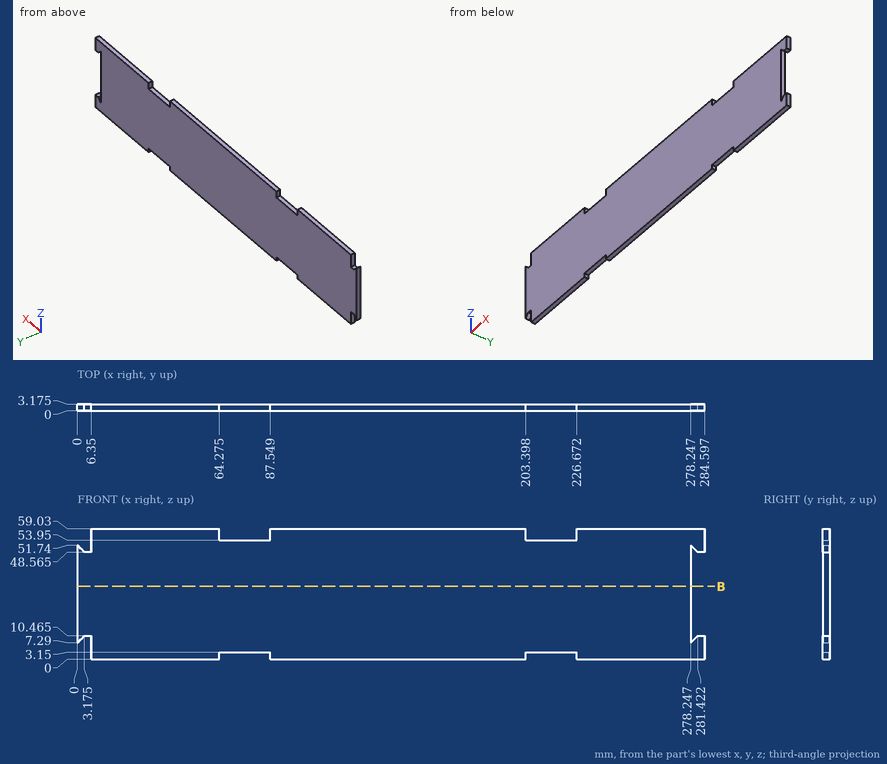
Could you check a few things on this drawing? It's one solid part, dimensions in mm from its lowest x, y, z. Coordinates: 2 decimals unless noted, no trailing zeros. Loops run counter-clockwise (first coordinate to the right, second up) from the corner with the lowest first, then second, coordinate; pieces in that order, holes last. Notation, with made-up numbers: (-14.5, 67) - (10.5, 67) arc R14 cw to (10.5, 79) - close; hole circle Ø11 at (40, 33.5). An arc over 180 degrees is marked (long way). Answer as a JSON object with one key per item and string values. Group by question number.
Item 1: For pin 1 (1 mm diameter, centred on x = 5.5, y = 1, fed in from +Z) (1 decimal); pin 2 (1 mm diameter, centred on y = 1, z = 55, fed in from -X); pin 3 (1.6 mm diameter, centred on x = 5, y = 2, fed in from -Z) (1 decimal), each with a flat end and sliding along its axis, tell me the tip position at first contact or that it passes through.
Item 2: If I drill on L1, parallel to X at y = 2.5, z = 12.5; L2, parallel to X at y = 0.35, z = 6; L3, parallel to Z at x = 204, y = 2.9, over which ranges is the centre line in solid material (lowest first)? Write a range as from..to.
Item 3: If we section it at B-B (z = 33): List the corners of the cut face in (x, y) for me (1 decimal).
Returned:
{
 "1": {"pin 1": "stops at z = 48.6", "pin 2": "stops at x = 6.35", "pin 3": "stops at z = 10.5"},
 "2": {"L1": "x = 0..278.25", "L2": "x = 6.35..284.6", "L3": "z = 3.15..53.95"},
 "3": {"outline": "(0, 0) - (278.2, 0) - (278.2, 3.2) - (0, 3.2) - close"}
}
